Input: dimensioned drawing with shaded views. Units: mm. Origin: part minimum x, y, z. A direction names the side the tool comes from. Round coordinates to 2 decimals unless told otherwise and drop trailing zeros. Write each loop counter-clockwise with the first axis right and the second up, starting at its lowest first coordinate (ties: lowest second). Pieces come first, ordered by that corner, then holes. Notation, with made-up numbers: M 65.25,39.25 L 121.25,39.25 A10 ccw 121.25,53.25 Z; hole C -8,42.5 d11. An arc over 180 degrees is marked long. Answer as CSV lines item,"result". Start each with the question number.
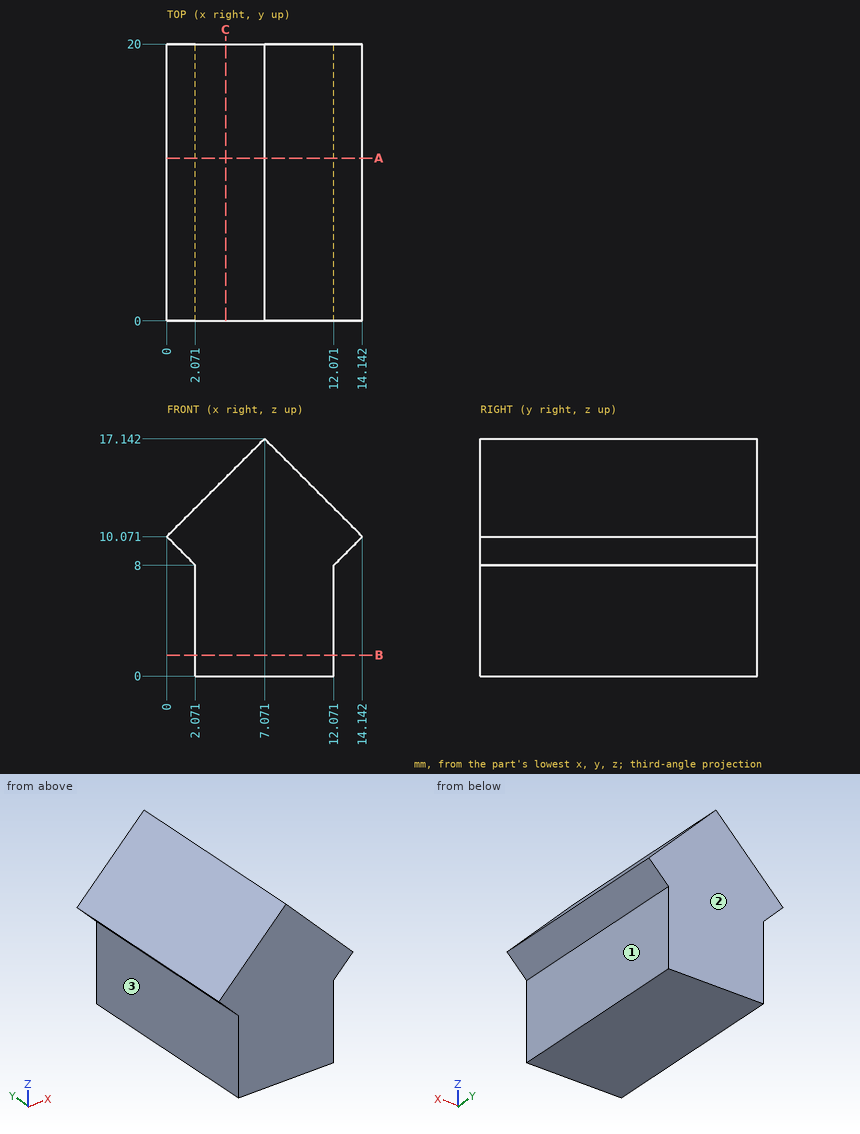
Item 1: Cut plane B-B, the plane z = 1.5. Return loops of the section in (x, y).
Item 2: Access query for the marked faces 1, 2 and 3. Directions: +Z, -Z, +X, -X, +Y, -Y. A direction counts if a zero-diameter tool reaches every point of the face in a straight line with its end or side. Return the directions, or none.
Item 3: Cut plane C-C, the plane x = 4.25. Return loops of the section in (y, z), plus the area to 3 significant figures.
Item 4: Pin query (flat end, axial travel): pin 1 Ø1.5 at (y, z) = (14, 5) entering from +X; pin 2 Ø1 at (x, y) = (12.5, 12.5) entering from +Z. Return the tip coordinate at first contact, or that it passes through.
Item 5: Line query: line 1 (X direction, y = 11.75, z = 2.25); line 2 (Z direction, x = 4.25, y = 18.25); line 3 (Z direction, x = 11.75, y = 4.25). Output: solid intervals per line, ascending. Write a range as [from, to].
Item 6: Cut plane A-A, the plane y = 11.75. Return loops of the section in (x, z).
Results list:
1,outline,"M 2.07,0 L 12.07,0 L 12.07,20 L 2.07,20 Z"
2,face 1,"-Z, +X, +Y, -Y"
2,face 2,"+Z, -Z, +X, -X, +Y"
2,face 3,"-Z, -X, +Y, -Y"
3,outline,"M 0,0 L 20,0 L 20,14.32 L 0,14.32 Z"
3,area,"286 mm²"
4,pin 1,"x = 12.07"
4,pin 2,"z = 12.21"
5,line 1,"[2.07, 12.07]"
5,line 2,"[0, 14.32]"
5,line 3,"[0, 12.46]"
6,outline,"M 0,10.07 L 2.07,8 L 2.07,0 L 12.07,0 L 12.07,8 L 14.14,10.07 L 7.07,17.14 Z"
